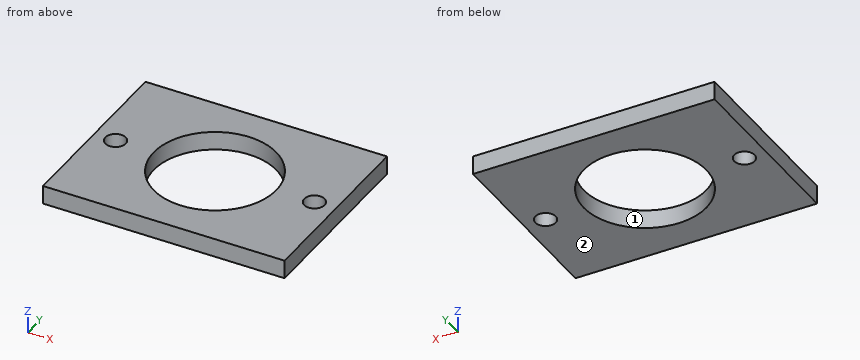
```python
from build123d import *

# Parameters (mm, degrees)
CAP_PLATE_26X20X2_START       = 7.2
CAP_PLATE_26X20X2_PROFILE_W   = 26
CAP_PLATE_26X20X2_PROFILE_H   = 20
CAP_PLATE_26X20X2_PROFILE_R   = 6.6
CAP_PLATE_26X20X2_PROFILE_R_2 = 1.1
CAP_PLATE_26X20X2_DEPTH       = 2


with BuildPart() as part:
    # Cap_plate_26x20x2_Profile → Cap_plate_26x20x2 (new body)
    with BuildSketch(Plane.XY.offset(CAP_PLATE_26X20X2_START)):
        with Locations((12.5, 0)):
            Rectangle(CAP_PLATE_26X20X2_PROFILE_W, CAP_PLATE_26X20X2_PROFILE_H)
        with Locations((12.5, 0)):
            Circle(CAP_PLATE_26X20X2_PROFILE_R, mode=Mode.SUBTRACT)
        with Locations((1.8, 0)):
            Circle(CAP_PLATE_26X20X2_PROFILE_R_2, mode=Mode.SUBTRACT)
        with Locations((23.2, 0)):
            Circle(CAP_PLATE_26X20X2_PROFILE_R_2, mode=Mode.SUBTRACT)
    extrude(amount=CAP_PLATE_26X20X2_DEPTH)


solid = part.part
```
Geometry check sheet. Reference: the model listing, model coordinates, mm. Face numbers are marked on the shaded views. Give positions to 0.01 mm unless a question says otherwise; leave off trailing zeros. Write each loop counter-clockwise with the first axis right and the second up, starting at its lowest first coordinate (ties: lowest second). Pieces come first, ordered by that corner, then holes. Notation, with made-up numbers: (-2, 13) -> (53, 13) arc R14 ccw to (53, 26) -> close; hole circle Ø4 at (73.25, -19.5). An arc over 180 degrees is marked (long way). One line per question, with ' | ' between items.
Item 1: Sectioned sample at B-B, the plane x = 23.2. Record the boundary of the cut face in (y, z), plus the area to 3 significant figures.
Determined:
outline: (-10, 7.2) -> (-1.1, 7.2) -> (-1.1, 9.2) -> (-10, 9.2) -> close; (1.1, 7.2) -> (10, 7.2) -> (10, 9.2) -> (1.1, 9.2) -> close | area: 35.6 mm^2
Item 2: Sectioned sample at D-D, the plane x = 12.5. Record the boundary of the cut face in (y, z).
Determined:
outline: (-10, 7.2) -> (-6.6, 7.2) -> (-6.6, 9.2) -> (-10, 9.2) -> close; (6.6, 7.2) -> (10, 7.2) -> (10, 9.2) -> (6.6, 9.2) -> close
Item 3: Sectioned sample at A-A, the plane y = 0. Record the boundary of the cut face in (x, z).
Determined:
outline: (-0.5, 7.2) -> (0.7, 7.2) -> (0.7, 9.2) -> (-0.5, 9.2) -> close; (2.9, 7.2) -> (5.9, 7.2) -> (5.9, 9.2) -> (2.9, 9.2) -> close; (19.1, 7.2) -> (22.1, 7.2) -> (22.1, 9.2) -> (19.1, 9.2) -> close; (24.3, 7.2) -> (25.5, 7.2) -> (25.5, 9.2) -> (24.3, 9.2) -> close
Item 4: Sectioned sample at C-C, the plane z = 8.9. Record the boundary of the cut face in (x, y), plus the area to 3 significant figures.
Determined:
outline: (-0.5, -10) -> (25.5, -10) -> (25.5, 10) -> (-0.5, 10) -> close; hole circle Ø2.2 at (1.8, 0); hole circle Ø13.2 at (12.5, 0); hole circle Ø2.2 at (23.2, 0) | area: 376 mm^2
Item 5: Depth check by flat-ended pin: pin 1 (1.3 mm diameter, centred on x = 1.8, y = 0, fed in from +Z). Enter the tip coordinate at first touch or a pass-through.
Determined:
pin 1: through
Item 6: Draft check along X on the marked faces 1 and 2. Enter one of: released by +X, released by -X, zero draft, split by the parting line, or undercut.
Determined:
face 1: undercut | face 2: zero draft
Item 7: Scan lines: line 1 along Y through (x, z) = (23.2, 8.2); line 2 along Y through (x, z) = (12.5, 8.3); line 3 along X through (y, z) = (1, 7.8). Record each from-to range of solid material in increasing order.
Determined:
line 1: -10 to -1.1, 1.1 to 10 | line 2: -10 to -6.6, 6.6 to 10 | line 3: -0.5 to 1.34, 2.26 to 5.98, 19.02 to 22.74, 23.66 to 25.5
